Autodesk Inventor part; units mm, degrees
ref_plane "YZ Plane" through (0, 0, 0) normal (1, 0, 0) x (0, 1, 0)
ref_plane "XZ Plane" through (0, 0, 0) normal (0, 1, 0) x (-1, 0, 0)
ref_plane "XY Plane" through (0, 0, 0) normal (0, 0, 1) x (1, 0, 0)
sketch "Esboço1" plane through (0, 0, 0) normal (0, 1, 0) x (-1, 0, 0)
  line L0 (-19.4, -29.1) -> (19.4, -29.1)
  line L1 (21.4, -27.1) -> (21.4, 27.1)
  line L2 (19.4, 29.1) -> (-19.4, 29.1)
  line L3 (-21.4, 27.1) -> (-21.4, -27.1)
  line L4 (-21.4, -29.1) -> (21.4, 29.1) construction
  line L5 (21.4, -29.1) -> (-21.4, 29.1) construction
  circle A0 centre (17.05, 24.75) radius 1.35
  circle A1 centre (-17.05, 24.75) radius 1.35
  circle A2 centre (17.05, -24.75) radius 1.35
  circle A3 centre (-17.05, -24.75) radius 1.35
  arc A4 (21.4, 27.1) -> (19.4, 29.1) centre (19.4, 27.1) ccw
  arc A5 (-19.4, 29.1) -> (-21.4, 27.1) centre (-19.4, 27.1) ccw
  arc A6 (19.4, -29.1) -> (21.4, -27.1) centre (19.4, -27.1) ccw
  arc A7 (-21.4, -27.1) -> (-19.4, -29.1) centre (-19.4, -27.1) ccw
  point P0 (0, 0)
  dimension "d0" = 42.8
  dimension "d1" = 58.2
  dimension "d2" = 2.7
  dimension "d3" = 3
  dimension "d4" = 3
  dimension "d5" = 2.7
  dimension "d6" = 3
  dimension "d7" = 3
  dimension "d8" = 2
extrude "Extrusão1" add sketch "Esboço1" along normal blind 1.8
sketch "Esboço2" plane through (0, 1.8, 0) normal (0, 1, 0) x (1, 0, 0)
  line L0 (-21.4, 27.1) -> (-21.4, -27.1)
  arc A0 (-21.4, -27.1) -> (-19.4, -29.1) centre (-19.4, -27.1) ccw
  arc A1 (-19.4, 29.1) -> (-21.4, 27.1) centre (-19.4, 27.1) ccw
  line L1 (19.4, 29.1) -> (-19.4, 29.1)
  line L2 (-19.4, -29.1) -> (19.4, -29.1)
  arc A2 (19.4, -29.1) -> (21.4, -27.1) centre (19.4, -27.1) ccw
  line L3 (21.4, -27.1) -> (21.4, 27.1)
  arc A3 (21.4, 27.1) -> (19.4, 29.1) centre (19.4, 27.1) ccw
  line L4 (20.7322, -8.55) -> (13.2322, -8.55)
  line L5 (13.2322, -8.55) -> (13.2322, 8.55)
  line L6 (13.2322, 8.55) -> (20.7322, 8.55)
  line L7 (20.7322, 8.55) -> (20.7322, -8.55)
  line L8 (20.7322, -8.55) -> (13.2322, 8.55) construction
  line L9 (13.2322, -8.55) -> (20.7322, 8.55) construction
  line L10 (20.7322, 10.1228) -> (13.2322, 10.1228)
  line L11 (13.2322, 10.1228) -> (13.2322, 20.1228)
  line L12 (13.2322, 20.1228) -> (20.7322, 20.1228)
  line L13 (20.7322, 20.1228) -> (20.7322, 10.1228)
  line L14 (-20.8142, -19.6445) -> (-6.7142, -19.6445)
  line L15 (-6.7142, -19.6445) -> (-6.7142, -12.8445)
  line L16 (-6.7142, -12.8445) -> (-20.8142, -12.8445)
  line L17 (-20.8142, -12.8445) -> (-20.8142, -19.6445)
  line L18 (-28.189, 0) -> (33.4078, 0)
  line L19 (-21.4, -2.2988) -> (-18.0103, -2.2988)
  line L20 (-18.0103, -2.2988) -> (-18.0103, 2.2923)
  line L21 (-18.0103, 2.2923) -> (-21.4, 2.2923)
  line L22 (-21.4, 2.2923) -> (-21.4, -2.2988)
  line L23 (-13.7642, -27.1) -> (0, -27.1)
  line L24 (0, -21.4359) -> (-13.7642, -21.4359)
  line L25 (-13.7642, -21.4359) -> (-13.7642, -27.1)
  line L26 (0, -28.5142) -> (11.7075, -28.5142)
  line L27 (11.7075, -28.5142) -> (11.7075, -19.6445)
  line L28 (11.7075, -19.6445) -> (0, -19.6445)
  line L29 (0, -19.6445) -> (0, -21.4359)
  line L30 (0, -27.1) -> (0, -28.5142)
  line L31 (-13.7642, 27.1) -> (0, 27.1)
  line L32 (0, 21.4359) -> (-13.7642, 21.4359)
  line L33 (-13.7642, 21.4359) -> (-13.7642, 27.1)
  line L34 (0, 28.5142) -> (11.7075, 28.5142)
  line L35 (11.7075, 28.5142) -> (11.7075, 19.6445)
  line L36 (11.7075, 19.6445) -> (0, 19.6445)
  line L37 (0, 19.6445) -> (0, 21.4359)
  line L38 (0, 27.1) -> (0, 28.5142)
  line L39 (3.5052, -8.55) -> (7.8476, -8.55)
  line L40 (7.8476, -8.55) -> (7.8476, -1.4997)
  line L41 (7.8476, -1.4997) -> (3.5052, -1.4997)
  line L42 (3.5052, -1.4997) -> (3.5052, -8.55)
  circle A4 centre (0, -5.0249) radius 3.428
  line L43 (-3.428, -18.1455) -> (0.572, -18.1455)
  line L44 (0.572, -18.1455) -> (0.572, -14.1455)
  line L45 (0.572, -14.1455) -> (-3.428, -14.1455)
  line L46 (-3.428, -14.1455) -> (-3.428, -18.1455)
  line L47 (-4.8578, 12.5931) -> (-0.8578, 12.5931)
  line L48 (-0.8578, 12.5931) -> (-0.8578, 16.5931)
  line L49 (-0.8578, 16.5931) -> (-4.8578, 16.5931)
  line L50 (-4.8578, 16.5931) -> (-4.8578, 12.5931)
  line L51 (1.8165, 12.5931) -> (5.8165, 12.5931)
  line L52 (5.8165, 12.5931) -> (5.8165, 16.5931)
  line L53 (5.8165, 16.5931) -> (1.8165, 16.5931)
  line L54 (1.8165, 16.5931) -> (1.8165, 12.5931)
  line L55 (-20.8142, 9.2758) -> (-18.3142, 9.2758)
  line L56 (-18.3142, 9.2758) -> (-18.3142, 16.2758)
  line L57 (-18.3142, 16.2758) -> (-20.8142, 16.2758)
  line L58 (-20.8142, 16.2758) -> (-20.8142, 9.2758)
  point P0 (0, 0)
  point P1 (16.9822, 0)
  dimension "d11" = 7.5
  dimension "d12" = 17.1
  dimension "d13" = 7.5
  dimension "d14" = 10
  dimension "d15" = 14.1
  dimension "d16" = 6.8
  dimension "d17" = 4
  dimension "d18" = 4
  dimension "d19" = 4
  dimension "d20" = 4
  dimension "d21" = 4
  dimension "d22" = 4
  dimension "d23" = 2.5
  dimension "d24" = 7
extrude "Extrusão2" add sketch "Esboço2" along normal blind 8.5 contours L18 L7 L4 L5 | L5 L6 L7 L18
extrude "Extrusão3" add sketch "Esboço2" along normal blind 10 contours L10 L11 L12 L13 | L17 L16 L15 L14
extrude "Extrusão4" add sketch "Esboço2" along normal blind 5.8 contours L25 L24 L29 L28 L27 L26 L30 L23 | L31 L38 L34 L35 L36 L37 L32 L33
extrude "Extrusão5" add sketch "Esboço2" along normal blind 1 contours L46 L45 L44 L43 | L50 L49 L48 L47 | L54 L53 L52 L51
extrude "Extrusão6" add sketch "Esboço2" along normal blind 2 contours L21 L20 L18 L0 | L18 L20 L19 L0 | L42 L41 L40 L39
extrude "Extrusão7" add sketch "Esboço2" along normal blind 9 contours L58 L57 L56 L55
extrude "Extrusão8" add sketch "Esboço2" along normal blind 6 contours A4
chamfer "Chanfro1" distance 2 angle 45 2 edges at (20.7322, 11.8, -15.1228) (13.2322, 11.8, -15.1228)
fillet "Arredondamento1" radius 1 4 edges at (20.7322, 10.3, 0) (13.2322, 10.3, 0) (16.9822, 10.3, 8.55) (16.9822, 10.3, -8.55)
fillet "Arredondamento2" radius 1 3 edges at (-13.7642, 11.8, 19.6445) (-13.7642, 11.8, 12.8445) (-6.7142, 11.8, 16.2445)
sketch "Esboço3" plane through (0, 3.8, 0) normal (0, 1, 0) x (1, 0, 0)
  line L0 (7.8476, -1.4997) -> (3.5052, -1.4997)
  line L1 (3.5052, -1.4997) -> (3.5052, -8.55)
  line L2 (7.8476, -8.55) -> (7.8476, -1.4997)
  line L3 (3.5052, -8.55) -> (7.8476, -8.55)
  line L4 (3.5052, -1.4997) -> (7.8476, -1.4997)
  line L5 (7.8476, -1.4997) -> (7.8476, -3.7821)
  line L6 (7.8476, -3.7821) -> (3.5052, -3.7821)
  line L7 (3.5052, -3.7821) -> (3.5052, -1.4997)
  line L8 (3.5052, -3.7821) -> (7.8476, -3.7821)
  line L9 (7.8476, -3.7821) -> (7.8476, -6.0999)
  line L10 (7.8476, -6.0999) -> (3.5052, -6.0999)
  line L11 (3.5052, -6.0999) -> (3.5052, -3.7821)
  line L12 (5.6764, -1.4997) -> (5.6764, -8.55)
  circle A0 centre (4.673, -2.6409) radius 0.5
  circle A1 centre (6.8599, -2.6409) radius 0.5
  circle A2 centre (4.673, -4.941) radius 0.5
  circle A3 centre (6.8599, -4.941) radius 0.5
  circle A4 centre (4.673, -7.5205) radius 0.5
  circle A5 centre (6.8599, -7.5205) radius 0.5
  point P0 (0, 0)
  dimension "d44" = 1
  dimension "d45" = 1
  dimension "d46" = 1
  dimension "d47" = 1
  dimension "d48" = 1
  dimension "d49" = 1
extrude "Extrusão9" add sketch "Esboço3" along normal blind 6 contours A0 | A1 | A2 | A3 | A4 | A5
sketch "Esboço4" plane through (0, 10.3, 0) normal (0, 1, 0) x (1, 0, 0)
  line L0 (14.2322, 7.55) -> (19.7322, 7.55)
  line L1 (14.2322, -7.55) -> (14.2322, 7.55)
  line L2 (19.7322, 7.55) -> (19.7322, -7.55)
  line L3 (19.7322, -7.55) -> (14.2322, -7.55)
  line L4 (18.8699, -6.7178) -> (15.0945, -6.7178)
  line L5 (15.0945, -6.7178) -> (15.0945, 6.7178)
  line L6 (15.0945, 6.7178) -> (18.8699, 6.7178)
  line L7 (18.8699, 6.7178) -> (18.8699, -6.7178)
  line L8 (18.8699, -6.7178) -> (15.0945, 6.7178) construction
  line L9 (15.0945, -6.7178) -> (18.8699, 6.7178) construction
  line L10 (15.0945, -2.2873) -> (18.8699, -2.2873)
  line L11 (18.8699, -2.2873) -> (18.8699, -6.7178)
  line L12 (18.8699, -6.7178) -> (15.0945, -6.7178)
  line L13 (15.0945, -6.7178) -> (15.0945, -2.2873)
  point P0 (0, 0)
  point P1 (16.9822, 0)
extrude "Extrusão10" add sketch "Esboço4" along normal blind 3 contours L4 L5 L10 L7
extrude "Extrusão11" cut sketch "Esboço4" against normal blind 0.5 contours L10 L5 L6 L7
fillet "Arredondamento3" radius 0.5 4 edges at (16.9822, 13.3, 6.7178) (18.8699, 13.3, 4.5025) (16.9822, 13.3, 2.2873) (15.0945, 13.3, 4.5025)
properties part number "SERIAL_BUS_SERVO_CONTROLLER"
Check sheet for the modelled part. Datum: model origin and axes. Units: mm. A direction names the side the tool comes from. Coordinates: 2 decimals unless noted, no trailing zeros. Order: outer loops, then holes, each group sorted by start corner. A loop starts at its lowest first (then second) coordinate and runs counter-clockwise, first axis right, second up. Notation, with made-up numbers: (1.25, 56.25) -> (22.25, 56.25) arc R29 cw to (22.25, 95.25) -> close; hole circle Ø8 at (71.25, 75). An arc over 180 degrees is marked (long way). Write item = value, one per line. Start each with the question number.
1) Access from +Z, -Z, +X, -X, +Y, -Y to the whole of each face (thin tool, end or side, straight path). Record for faces 1 (the flat face through (-7, 5, -21.436)), 2 (the flat face through (20.732, 5, 0)), 3 (the flat face through (6, 3, 8.55)), 4 (the flat face through (-1, 7.6, 24)).
2) Material ranges on L1, parallel to Z at x = 17.05, y = 0.55; L2, parallel to Z at x = -3, y = 6.5; L3, parallel to Z at x = -6, y = 6.25, recorded low to high.
3) Go/stop test with flat-tipped pins: P1, Ø4, axis at y = 10, z = 16.5, coming from the +X side; P2, Ø2, axis at x = 16.5, y = 5, coming from the +Z side; P3, Ø2, axis at x = 17, y = 4.5, coming from the -Z side. Record where each tip stops, or that it passes through.
4) Cross-section at D-D (y = 5.5). State how many separate pieces and enclosed holes the cut face has, then the cut area to 3 significant figures.
5) Cross-section at B-B (z = 24.75). Enter the section's corners in (x, y).
6) Cross-section at C-C (z = 16). Enter the section's corners in (x, y), then the cut area to 3 significant figures.
7) Mould release check, pull along Z, two halves, no side actions. Record for faces 5 (the flat face through (-20, 10.8, -13)), 6 (the flat face through (-7, 5, 21.436)), 7 (the flat face through (6, 5, -28.514)), 8 (the cylindrical face through (15.803, 0.887, -24.233)): +Z half, -Z half, draft (parallel to the pull), parting line (faces both ways), or undercut.
8) Cross-section at A-A (x = -17.05). Enter the section's corners in (y, z).
Ans:
q1.face_1 = -X, +Y
q1.face_2 = +Z, -Z, +X, +Y
q1.face_3 = +X, -X, +Y
q1.face_4 = +Z, +X, -X, +Y
q2.L1 = -29.1 to -26.1, -23.4 to 23.4, 26.1 to 29.1
q2.L2 = -27.1 to -21.44, 3.37 to 6.68, 21.44 to 27.1
q2.L3 = -27.1 to -21.44, 21.44 to 27.1
q3.P1 = -6.71
q3.P2 = 8.55
q3.P3 = -20.12
q4.separate_pieces = 13
q4.enclosed_holes = 0
q4.area = 722 mm²
q5.outline = (-21.4, 0) -> (-18.4, 0) -> (-18.4, 1.8) -> (-21.4, 1.8) -> close; (-15.7, 0) -> (15.7, 0) -> (15.7, 1.8) -> (11.71, 1.8) -> (11.71, 7.6) -> (-13.76, 7.6) -> (-13.76, 1.8) -> (-15.7, 1.8) -> close; (18.4, 0) -> (21.4, 0) -> (21.4, 1.8) -> (18.4, 1.8) -> close
q6.outline = (-21.4, 0) -> (21.4, 0) -> (21.4, 1.8) -> (0.57, 1.8) -> (0.57, 2.8) -> (-3.43, 2.8) -> (-3.43, 1.8) -> (-6.71, 1.8) -> (-6.71, 10.8) arc R1 ccw to (-7.71, 11.8) -> (-20.81, 11.8) -> (-20.81, 1.8) -> (-21.4, 1.8) -> close
q6.area = 222 mm²
q7.face_5 = draft
q7.face_6 = undercut
q7.face_7 = -Z half
q7.face_8 = undercut
q8.outline = (0, -29.1) -> (1.8, -29.1) -> (1.8, -26.1) -> (0, -26.1) -> close; (0, -23.4) -> (1.8, -23.4) -> (1.8, 12.84) -> (10.8, 12.84) arc R1 ccw to (11.8, 13.84) -> (11.8, 18.64) arc R1 ccw to (10.8, 19.64) -> (1.8, 19.64) -> (1.8, 23.4) -> (0, 23.4) -> close; (0, 26.1) -> (1.8, 26.1) -> (1.8, 29.1) -> (0, 29.1) -> close
